Part model, mm, in its own coordinate system. Give positions to 0.01 mm unless a question says otherwise; leave off trailing zeros. Write each loop counter-clockwise with the first axis right and the second up, starting at its lowest first coordinate (ties: lowest second). Pieces come first, ordered by that corner, then holes. Notation, with made-up numbers: M -1.75,66 L 34.25,66 A26 cw 34.25,103 Z; hole C 0,76 d1. An arc over 180 degrees is marked long. Use CSV: the item, a comma, the result in double quotes. Start each with the question number.
Item 1: Pin check, flat tips, straight feed: pin 1 (4 mm diameter, centred on x = 37.4, y = 7.5, fed in from -Z); pin 2 (2 mm diameter, centred on x = 9.9, y = 10.85, fed in from +Z); pin 3 (0.8 mm diameter, centred on y = 9, z = 1.5, fed in from +X). Stop position of each tip, or through.
Item 2: Cut at C-C (z = 1.9). List the corners of the cut face in (x, y).
Item 3: Cut at A-A (y = 7.5). List the corners of the cut face in (x, z), then the cut area to 4 significant figures.
Item 4: Cut at D-D (x = 37.4). List the corners of the cut face in (y, z), then the cut area to 3 significant figures.
Item 5: Drill centre lines: line 1 (X direction, y = 7, z = 1.75); line 2 (Y direction, x = 30.9, z = 0.85); line 3 (Y direction, x = 47.5, z = 2.05). Where is each one in solid material? Low to high. Write a range as [from, to].
Item 6: Cut at B-B (x = 9.9). List the corners of the cut face in (y, z).
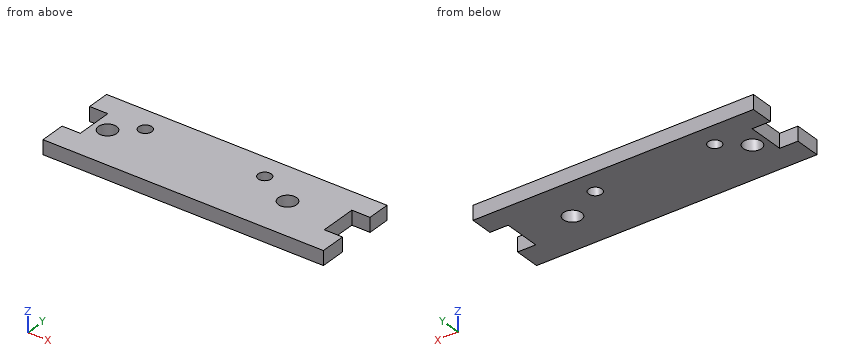
from build123d import *

# Parameters (mm, degrees)
SKETCH_1_W          = 49.3
SKETCH_1_H          = 15
EXTRUDE_1_DEPTH     = 2.5
SKETCH_2_R          = 1.6
CUT_EXTRUDE_1_DEPTH = 52.592053652
SKETCH_3_W          = 3.2
SKETCH_3_H          = 6.5
CUT_EXTRUDE_2_DEPTH = 10
SKETCH_4_R          = 1.15
CUT_EXTRUDE_3_DEPTH = 10


with BuildPart() as part:
    # 草图1 → 凸台-拉伸1 (new body)
    with BuildSketch(Plane.XY):
        with Locations((24.65, 7.5)):
            Rectangle(SKETCH_1_W, SKETCH_1_H)
    extrude(amount=EXTRUDE_1_DEPTH)

    # 草图2 → 切除-拉伸1 (cut, through all)
    with BuildSketch(Plane(origin=(0, 0, 0), x_dir=(-1, 0, 0), z_dir=(0, 0, -1))):
        with Locations((-5.75, 7.5)):
            Circle(SKETCH_2_R)
        with Locations((-37.4, 7.5)):
            Circle(SKETCH_2_R)
    extrude(amount=-CUT_EXTRUDE_1_DEPTH, mode=Mode.SUBTRACT)

    # 草图3 → 切除-拉伸2 (cut)
    with BuildSketch(Plane.XY.offset(2.5)):
        with Locations((1.6, 7.75)):
            Rectangle(SKETCH_3_W, SKETCH_3_H)
    cut_extrude_2 = extrude(amount=-CUT_EXTRUDE_2_DEPTH, mode=Mode.SUBTRACT)

    # 镜向1: 切除-拉伸2 across plane
    add(cut_extrude_2.mirror(Plane.ZY.offset(-24.65)), mode=Mode.SUBTRACT)

    # 草图4 → 切除-拉伸3 (cut)
    with BuildSketch(Plane.XY.offset(2.5)):
        with Locations((9.9, 10.85)):
            Circle(SKETCH_4_R)
        with Locations((30.9, 10.85)):
            Circle(SKETCH_4_R)
    extrude(amount=-CUT_EXTRUDE_3_DEPTH, mode=Mode.SUBTRACT)


solid = part.part
Worked answers:
1,pin 1,"stops at z = 0"
1,pin 2,"passes through"
1,pin 3,"stops at x = 46.1"
2,outline,"M 0,0 L 49.3,0 L 49.3,4.5 L 46.1,4.5 L 46.1,11 L 49.3,11 L 49.3,15 L 0,15 L 0,11 L 3.2,11 L 3.2,4.5 L 0,4.5 Z; hole C 5.75,7.5 d3.2; hole C 9.9,10.85 d2.3; hole C 30.9,10.85 d2.3; hole C 37.4,7.5 d3.2"
3,outline,"M 3.2,0 L 4.15,0 L 4.15,2.5 L 3.2,2.5 Z; M 7.35,0 L 35.8,0 L 35.8,2.5 L 7.35,2.5 Z; M 39,0 L 46.1,0 L 46.1,2.5 L 39,2.5 Z"
3,area,"91.25 mm^2"
4,outline,"M 0,0 L 5.9,0 L 5.9,2.5 L 0,2.5 Z; M 9.1,0 L 15,0 L 15,2.5 L 9.1,2.5 Z"
4,area,"29.5 mm^2"
5,line 1,"x = [3.2, 4.23], [7.27, 35.88], [38.92, 46.1]"
5,line 2,"y = [0, 9.7], [12, 15]"
5,line 3,"y = [0, 4.5], [11, 15]"
6,outline,"M 0,0 L 9.7,0 L 9.7,2.5 L 0,2.5 Z; M 12,0 L 15,0 L 15,2.5 L 12,2.5 Z"
